```python
from build123d import *

# Parameters (mm, degrees)
SKETCH_1_W          = 50
SKETCH_1_H          = 50
SKETCH_1_R          = 21
EXTRUDE_1_DEPTH     = 3
SKETCH_2_W          = 50
SKETCH_2_H          = 30
SKETCH_2_R          = 1.45
EXTRUDE_2_DEPTH     = 3
FILLET_1_R          = 3
SKETCH_3_R          = 1.45
CUT_EXTRUDE_1_DEPTH = 61.489668539
CUT_EXTRUDE_7_DEPTH = 61.489668539
SKETCH_13_W         = 6
SKETCH_13_H         = 17.5
EXTRUDE_3_DEPTH     = 3
FILLET_2_R          = 2


with BuildPart() as part:
    # 草图1 → 凸台-拉伸1 (new body)
    with BuildSketch(Plane(origin=(0, 0, 0), x_dir=(1, 0, 0), z_dir=(0, 1, 0))):
        Rectangle(SKETCH_1_W, SKETCH_1_H)
        with Locations(Location((0, 0, 0), (0, 0, 270))):
            Circle(SKETCH_1_R, mode=Mode.SUBTRACT)
    extrude(amount=EXTRUDE_1_DEPTH)

    # 草图2 → 凸台-拉伸2 (add)
    with BuildSketch(Plane(origin=(0, 3, 0), x_dir=(1, 0, 0), z_dir=(0, 1, 0))):
        with Locations((0, -40)):
            Rectangle(SKETCH_2_W, SKETCH_2_H)
        with Locations(Location((-15, -47.5, 0), (0, 0, 270))):
            Circle(SKETCH_2_R, mode=Mode.SUBTRACT)
        with Locations(Location((15, -47.5, 0), (0, 0, 270))):
            Circle(SKETCH_2_R, mode=Mode.SUBTRACT)
    extrude(amount=-EXTRUDE_2_DEPTH)

    # 圆角1
    fillet_1_edges = [part.edges().sort_by_distance(p)[0] for p in [
        (25, 1.5, 55),
        (-25, 1.5, 55),
        (-25, 1.5, -25),
        (25, 1.5, -25),
    ]]
    fillet(fillet_1_edges, radius=FILLET_1_R)

    # 草图3 → 切除-拉伸1 (cut, through all)
    with BuildSketch(Plane(origin=(0, 3, 0), x_dir=(1, 0, 0), z_dir=(0, 1, 0))):
        with Locations(Location((-15, -30, 0), (0, 0, 270))):
            Circle(SKETCH_3_R)
        with Locations(Location((15, -30, 0), (0, 0, 270))):
            Circle(SKETCH_3_R)
    extrude(amount=-CUT_EXTRUDE_1_DEPTH, mode=Mode.SUBTRACT)

    # 草图12 → 切除-拉伸7 (cut, through all)
    with BuildSketch(Plane(origin=(0, 3, 0), x_dir=(1, 0, 0), z_dir=(0, 1, 0))):
        with BuildLine():
            ThreePointArc((-8.55, -30), (-10.439161261, -34.560838739), (-15, -36.45))
            Line((-15, -36.45), (-15, -41.05))
            ThreePointArc((-15, -41.05), (-10.439161261, -42.939161261), (-8.55, -47.5))
            Line((-8.55, -47.5), (8.55, -47.5))
            ThreePointArc((8.55, -47.5), (10.439161261, -42.939161261), (15, -41.05))
            Line((15, -41.05), (15, -36.45))
            ThreePointArc((15, -36.45), (10.439161261, -34.560838739), (8.55, -30))
            Line((8.55, -30), (-8.55, -30))
        make_face()
    extrude(amount=-CUT_EXTRUDE_7_DEPTH, mode=Mode.SUBTRACT)

    # 草图13 → 凸台-拉伸3 (add)
    with BuildSketch(Plane(origin=(0, 3, 0), x_dir=(1, 0, 0), z_dir=(0, 1, 0))):
        with Locations((0, -38.75)):
            Rectangle(SKETCH_13_W, SKETCH_13_H)
    extrude(amount=-EXTRUDE_3_DEPTH)

    # 圆角2
    fillet_2_edges = [part.edges().sort_by_distance(p)[0] for p in [
        (-3, 1.5, 30),
        (3, 1.5, 30),
        (3, 1.5, 47.5),
        (-3, 1.5, 47.5),
        (15, 1.5, 41.05),
        (8.55, 1.5, 47.5),
        (-8.55, 1.5, 47.5),
        (-15, 1.5, 41.05),
        (-15, 1.5, 36.45),
        (-8.55, 1.5, 30),
        (8.55, 1.5, 30),
        (15, 1.5, 36.45),
    ]]
    fillet(fillet_2_edges, radius=FILLET_2_R)


solid = part.part
```
Geometry: final body of the model. Coordinates: model frame, mm. A direction names the side the tool comes from. Round coordinates to 2 decimals unless told otherwise and drop trailing zeros. Write each loop counter-clockwise with the first axis right and the second up, starting at its lowest first coordinate (ties: lowest second). Pieces come first, ordered by that corner, then holes.
Item 1: Mould query, pull axis Z, two halves, no side actions, for faces 1 (the face through (0, 2, 55)), 2 (the face through (-24.14, 1.52, -24.1)), 3 (the face through (-3.6, 1.48, 46.93)). Classes: +Z half, -Z half, draft (parallel to the pull), parting line (faces both ways), or undercut.
Item 2: Section query D-D (y = 2.05). Give the number of separate pieces and of enclosed holes in the cut face, plus the area to 3 significant figures.
Item 3: Set-up query: faces 4 (the face through (25, 2, 16)), 5 (the face through (14.56, 1.48, 40.54)). Return all of +Z, -Z, +X, -X, +Y, -Y with unobstructed straight access to the full face (end or side cutting, diameter ignored); none if empty.
Item 4: Material intervals for L1, parallel to X at y = 1.7, z = 39; L2, parallel to Z at x = -13, y = 2.15; L3, parallel to Z at x = 10.5, y = 2.4, sorted ascending.
Item 5: Section query C-C (x = 9.5). Return loops of the section in (y, z), plus the area to 3 significant figures.
Item 6: Section query B-B (z = -1.5). Return loops of the section in (x, y).
Item 7: Section query A-A (x = 0). Return loops of the section in (y, z), plus the area to 3 significant figures.
Completed:
1. face 1: +Z half
1. face 2: -Z half
1. face 3: undercut
2. separate pieces: 1
2. enclosed holes: 7
2. area: 2,300 mm2
3. face 4: +Z, -Z, +X, +Y, -Y
3. face 5: +Y, -Y
4. L1: x = -25 to -15, -3 to 3, 15 to 25
4. L2: z = -25 to -16.49, 16.49 to 36.13, 41.37 to 55
4. L3: z = -25 to -18.19, 18.19 to 34.62, 42.88 to 55
5. outline: (0, -25) - (3, -25) - (3, -18.73) - (0, -18.73) - close; (0, 18.73) - (3, 18.73) - (3, 33.37) - (0, 33.37) - close; (0, 44.13) - (3, 44.13) - (3, 55) - (0, 55) - close
5. area: 95.3 mm2
6. outline: (-25, 0) - (-20.95, 0) - (-20.95, 3) - (-25, 3) - close; (20.95, 0) - (25, 0) - (25, 3) - (20.95, 3) - close
7. outline: (0, -25) - (3, -25) - (3, -21) - (0, -21) - close; (0, 21) - (3, 21) - (3, 55) - (0, 55) - close
7. area: 114 mm2
